from build123d import *

# Parameters (mm, degrees)
F0_W     = 327
F0_H     = 322
F1_DEPTH = 16.5
F2_T     = -6
F3_W     = 165
F3_H     = 160
F4_DEPTH = 16.501
F6_D     = 14


with BuildPart() as f1:
    # F0 (on Top) → F1 (new body, symmetric)
    with BuildSketch(Plane.XY):
        Rectangle(F0_W, F0_H)
    extrude(amount=F1_DEPTH, both=True)

    # F2
    f2_openings = [f1.faces().sort_by_distance(p)[0] for p in [
        (0, 0, 16.5),
    ]]
    offset(amount=F2_T, openings=f2_openings)

    # F3 (on Top) → F4 (cut, through all)
    with BuildSketch(Plane.XY):
        Rectangle(F3_W, F3_H)
    extrude(amount=-F4_DEPTH, mode=Mode.SUBTRACT)

    # F6 (through all)
    with Locations(Plane.XY.offset(-10.5)):
        with Locations((-135, 130), (135, 130), (135, -130), (-135, -130)):
            Hole(F6_D / 2)


solid = f1.part
Can you work these out from the model? Positions are in its coordinate system, mm. A direction names the side the tool comes from. Round coordinates to 2 decimals unless told otherwise and drop trailing zeros. Order: outer loops, then holes, each group sorted by start corner. A loop starts at its lowest first (then second) coordinate and runs counter-clockwise, first axis right, second up. Notation, with made-up numbers: (-37.5, 5) -> (5.5, 5) arc R21 ccw to (5.5, 13) -> close; hole circle Ø4 at (1.25, 57). An arc over 180 degrees is marked (long way). Write each question's results on one line, items separated by ' | '. Start each with the question number.
Item 1: Thinking about a two-plate mould opening in X: for faces 1 (the flat face through (-2, -105, -16.5)), 2 (the flat face through (163.5, -2, 0)), 3 (the cylindrical face through (140.16, 134.73, -13.54)), which applies, +X half, -X half, draft (parallel to the pull), parting line (faces both ways), or undercut?
Item 2: If we section it at C-C, the plane x = 27: Write out the boundary of the cut face in (y, z), then the cut area to 3 significant figures.
Item 3: Which directions (+Z, -Z, +X, -X, +Y, -Y) give clear straight access to the entire face, cutting with the end or side of a thin tool? Please do faces 4 (the flat face through (-2, 161, 0)), 5 (the flat face through (-2, 106, -10.5)).
Item 4: Please list where these lines run through material, in increasing order: L1, parallel to Y at x = -135, z = -15.1; L2, parallel to Y at x = 123.5, z = 3.5; L3, parallel to X at y = -91, z = -1.
Item 5: If we section it at A-A, the plane x = -135: Write out the boundary of the cut face in (y, z), then the cut area to 3 significant figures.
Item 6: If we section it at B-B, the plane y = -130: Write out the boundary of the cut face in (x, z).
Item 7: If we section it at D-D, the plane z = 11: Write out the boundary of the cut face in (x, y), then the cut area to 3 significant figures.
Results:
1) face 1: draft | face 2: +X half | face 3: undercut
2) outline: (-161, -16.5) -> (-80, -16.5) -> (-80, -10.5) -> (-155, -10.5) -> (-155, 16.5) -> (-161, 16.5) -> close; (80, -16.5) -> (161, -16.5) -> (161, 16.5) -> (155, 16.5) -> (155, -10.5) -> (80, -10.5) -> close | area: 1,300 mm2
3) face 4: +Z, -Z, +X, -X, +Y | face 5: +Z
4) L1: y = -161 to -137, -123 to 123, 137 to 161 | L2: y = -161 to -155, 155 to 161 | L3: x = -163.5 to -157.5, 157.5 to 163.5
5) outline: (-161, -16.5) -> (-137, -16.5) -> (-137, -10.5) -> (-155, -10.5) -> (-155, 16.5) -> (-161, 16.5) -> close; (-123, -16.5) -> (123, -16.5) -> (123, -10.5) -> (-123, -10.5) -> close; (137, -16.5) -> (161, -16.5) -> (161, 16.5) -> (155, 16.5) -> (155, -10.5) -> (137, -10.5) -> close | area: 2,090 mm2
6) outline: (-163.5, -16.5) -> (-142, -16.5) -> (-142, -10.5) -> (-157.5, -10.5) -> (-157.5, 16.5) -> (-163.5, 16.5) -> close; (-128, -16.5) -> (128, -16.5) -> (128, -10.5) -> (-128, -10.5) -> close; (142, -16.5) -> (163.5, -16.5) -> (163.5, 16.5) -> (157.5, 16.5) -> (157.5, -10.5) -> (142, -10.5) -> close
7) outline: (-163.5, -161) -> (163.5, -161) -> (163.5, 161) -> (-163.5, 161) -> close; hole (-157.5, -155) -> (157.5, -155) -> (157.5, 155) -> (-157.5, 155) -> close | area: 7,640 mm2
